Study the drawing (mm; zero at the part's minimum x, y, z) and answer. Coordinates: 2 decimals unless noted, no trailing zeros. Write each loop counter-clockwise with the first axis right and the second up, starting at its lowest first coordinate (ties: lowest second). Pieces come first, ordered by that corner, then holes. Notation, with made-up numbers: M -14.75,71.5 L 17.25,71.5 A22 ccw 17.25,89.5 Z; hole C -6.75,-6.5 d1. An arc over 180 degrees is marked long. Answer as CSV lines item,"result". Start each with the question number.
(1) A cutting plane is placed at C-C on y = 33. Give the vertices of the cut face in (x, z) (1 decimal).
(2) A cutting plane is placed at B-B on y = 50.8. Give the vertices of the cut face in (x, z).
(3) The mould has two halves that part along X. Classify the marked faces 1, 2, 3 and 4: released by +X, released by -X, zero draft, split by the parting line, or undercut.
(4) Flat-ended cylindrical pins translate along their axes: P1, Ø3, axis at x = 64, z = 9, coming from the -Y side (1 decimal); P2, Ø4, axis at y = 86, z = 3.5, coming from the -X side. Find the tip coordinate at first contact, or state that the pin passes through.
(5) A cutting plane is placed at A-A on x = 50.8. Give the vertices of the cut face in (y, z).
(6) Find the intervals of material crossed by L1, parallel to Y at x = 50.8, z = 3.25; L2, parallel to Y at x = 75.5, z = 8.75; L3, parallel to X at y = 39, z = 9.5 (1 decimal), in increasing order. Write a range as [from, to].
(7) A cutting plane is placed at D-D on x = 25.5. Give the vertices of the cut face in (y, z).
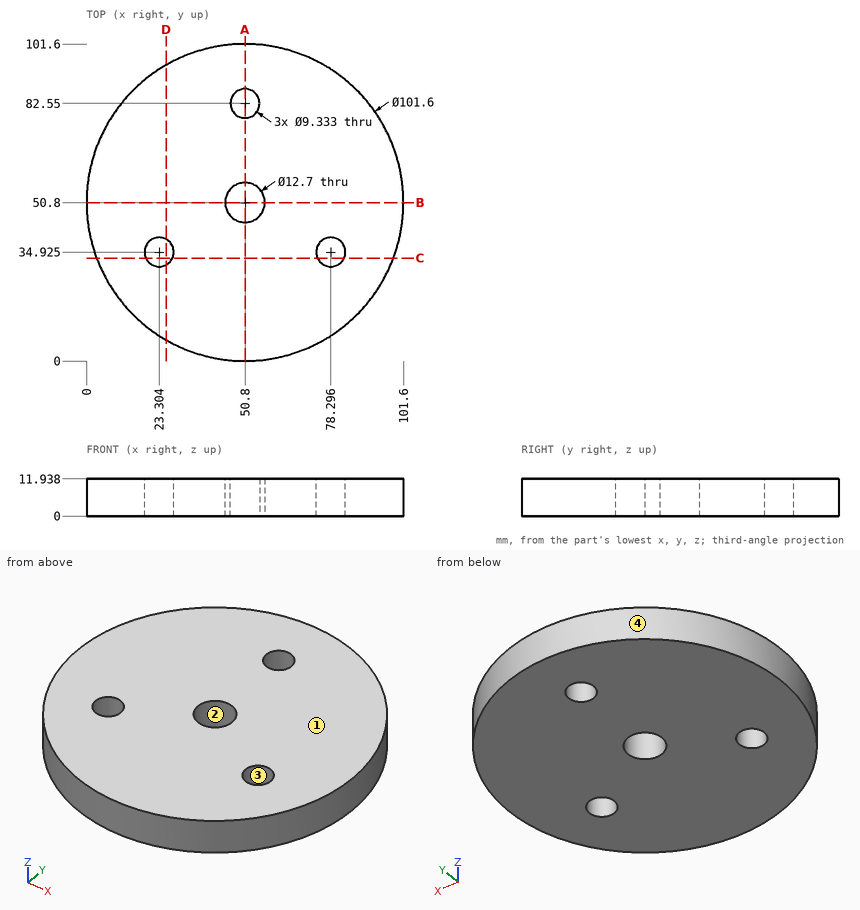
Here are the results:
1,outline,"M 3.2,0 L 19.1,0 L 19.1,11.9 L 3.2,11.9 Z; M 27.6,0 L 74,0 L 74,11.9 L 27.6,11.9 Z; M 82.5,0 L 98.4,0 L 98.4,11.9 L 82.5,11.9 Z"
2,outline,"M 0,0 L 44.45,0 L 44.45,11.94 L 0,11.94 Z; M 57.15,0 L 101.6,0 L 101.6,11.94 L 57.15,11.94 Z"
3,face 1,"zero draft"
3,face 2,"undercut"
3,face 3,"undercut"
3,face 4,"split by the parting line"
4,P1,"stops at y = 1.4"
4,P2,"stops at x = 12.35"
5,outline,"M 0,0 L 44.45,0 L 44.45,11.94 L 0,11.94 Z; M 57.15,0 L 77.88,0 L 77.88,11.94 L 57.15,11.94 Z; M 87.22,0 L 101.6,0 L 101.6,11.94 L 87.22,11.94 Z"
6,L1,"y = [0, 44.45], [57.15, 77.88], [87.22, 101.6]"
6,L2,"y = [6.41, 31.19], [38.66, 95.19]"
6,L3,"x = [1.4, 21], [25.6, 76], [80.6, 100.2]"
7,outline,"M 6.75,0 L 30.81,0 L 30.81,11.94 L 6.75,11.94 Z; M 39.04,0 L 94.85,0 L 94.85,11.94 L 39.04,11.94 Z"
